Part model, mm, in its own coordinate system. Face numbers are marked on the shaded views. A direction names the side the tool comes from. Coordinates: 2 decimals unless noted, no trailing zeros. Order: outer loops, then holes, each group sorted by start corner. A loop starts at its lowest first (then second) coordinate and runs counter-clockwise, first axis right, second up. Notation, with made-up numbers: M -30,40 L -17,40 A31 ccw -17,79 Z; hole C 88,73.25 d11. An arc over 180 degrees is marked long. Write item = value, one per line. Start each with the question number.
from build123d import *

# Parameters (mm, degrees)
BASE_FLANGE1_DEPTH      = 44
CUT_EXTRUDE1_DEPTH      = 57
CUT_EXTRUDE1_DEPTH_BACK = 42
SKETCH7_R               = 4
CUT_EXTRUDE2_DEPTH      = 42
SKETCH8_R               = 7.25
CUT_EXTRUDE3_DEPTH      = 42
SKETCH9_W               = 2.5
SKETCH9_H               = 6
CUT_EXTRUDE4_DEPTH      = 13


# Sheet-metal steps are written as plain solids
with BuildPart() as part:
    # Sketch1 → Base-Flange1 (new body)
    with BuildSketch(Plane.XY):
        with BuildLine():
            Line((15, 0), (15, 73.75))
            ThreePointArc((15, 73.75), (14.121320344, 75.871320344), (12, 76.75))
            Line((12, 76.75), (-12, 76.75))
            ThreePointArc((-12, 76.75), (-14.121320344, 75.871320344), (-15, 73.75))
            Line((-15, 73.75), (-15, 0))
            Line((-15, 0), (-17.3, 0))
            Line((-17.3, 0), (-17.3, 73.75))
            ThreePointArc((-17.3, 73.75), (-15.74766594, 77.49766594), (-12, 79.05))
            Line((-12, 79.05), (12, 79.05))
            ThreePointArc((12, 79.05), (15.74766594, 77.49766594), (17.3, 73.75))
            Line((17.3, 73.75), (17.3, 0))
            Line((17.3, 0), (15, 0))
        make_face()
    extrude(amount=BASE_FLANGE1_DEPTH)

    # Sketch6 → Cut-Extrude1 (cut, two sides: drawn at the far end of the back side and taken through both)
    with BuildSketch(Plane(origin=(0, 0, 0), x_dir=(0, 0, -1), z_dir=(1, 0, 0)).offset(-CUT_EXTRUDE1_DEPTH_BACK)):
        with BuildLine():
            Line((0, 73.75), (-24.610061631, 6.560660321))
            ThreePointArc((-24.610061631, 6.560660321), (-35.746513142, 0.153696539), (-44, 10))
            Line((-44, 10), (-44, 36.875))
            Line((-44, 36.875), (-75.735832134, 36.875))
            Line((-75.735832134, 36.875), (-75.735832134, -15.470238138))
            Line((-75.735832134, -15.470238138), (20.414497878, -15.470238138))
            Line((20.414497878, -15.470238138), (20.414497878, 73.75))
            Line((20.414497878, 73.75), (0, 73.75))
        make_face()
    extrude(amount=CUT_EXTRUDE1_DEPTH + CUT_EXTRUDE1_DEPTH_BACK, mode=Mode.SUBTRACT)

    # Sketch7 → Cut-Extrude2 (cut)
    with BuildSketch(Plane(origin=(17.3, 0, 0), x_dir=(0, 0, -1), z_dir=(1, 0, 0))):
        with Locations(Location((-34, 10, 0), (0, 0, 90))):
            Circle(SKETCH7_R)
    extrude(amount=-CUT_EXTRUDE2_DEPTH, mode=Mode.SUBTRACT)

    # Sketch8 → Cut-Extrude3 (cut)
    with BuildSketch(Plane(origin=(0, 79.05, 0), x_dir=(1, 0, 0), z_dir=(0, 1, 0))):
        with Locations(Location((0, -22, 0), (0, 0, 270))):
            Circle(SKETCH8_R)
    extrude(amount=-CUT_EXTRUDE3_DEPTH, mode=Mode.SUBTRACT)

    # Sketch9 → Cut-Extrude4 (cut)
    with BuildSketch(Plane.ZY.offset(17.3)):
        with Locations((34, 13)):
            Rectangle(SKETCH9_W, SKETCH9_H)
    extrude(amount=-CUT_EXTRUDE4_DEPTH, mode=Mode.SUBTRACT)


solid = part.part
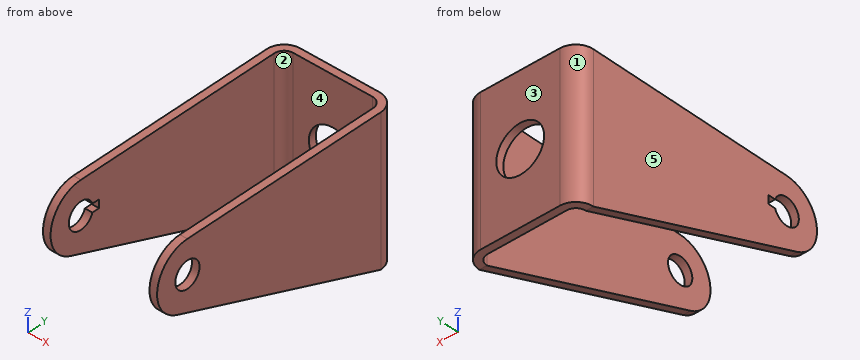
Item 1: 3-axis set-ups, long thin cutter, end or side, ignore diameter. For the marked faces 1 and 2: which of +Z, -Z, +X, -X, +Y, -Y reach the whole face in a straight line?
Item 2: Pull direction X, two halves, no side cores. Call the marked faces 3, 4 and 5: pulls with the +X half, pulls with the -X half, needs draft (parallel to the pull), parting line crosses it, or undercut.
Item 3: Wall check: line 1 along X through (y, z) = (37.5, 37.5); line 2 along Y through (x, z) = (8.5, 38.5); line 3 along Z through (x, y) = (-16.5, 10). Give the ranges that are in metal, low to high. Write a range as [from, to].
Item 4: Cut at D-D, the plane z = 22.5. Write the cut outline in (x, y).
Item 5: Cut at A-A, the plane x = 0. Write the cut outline in (y, z), and give its area (4 significant figures).
Item 6: Flat gauge pins, fed straight in: pin 1 (1.5 mm diameter, centred on x = 13, z = 6.5, fed in from -Y); pin 2 (0.7 mm diameter, centred on x = -16.5, y = 15, fed in from -Z); pin 3 (12 mm diameter, centred on x = -3.5, z = 20, fed in from -Y). Where does each tip first touch, or does it go through?
Item 7: Cut at B-B, the plane z = 34. Write the cut outline in (x, y), and give its area (3 significant figures).
Item 8: Cut at C-C, the plane y = 37. Write the cut outline in (x, z).
Filled sheet:
q1.face_1 = +Z, -Z, -X, +Y
q1.face_2 = +Z, -Z, -Y
q2.face_3 = needs draft
q2.face_4 = undercut
q2.face_5 = pulls with the -X half
q3.line_1 = [-17.3, -15], [15, 17.3]
q3.line_2 = [76.75, 79.05]
q3.line_3 = [23.35, 30], [38, 44]
q4.outline = M -17.3,12.32 L -15,12.32 L -15,73.75 A3 cw -12,76.75 L -7.23,76.75 L -7.23,79.05 L -12,79.05 A5.3 ccw -17.3,73.75 Z; M 7.23,76.75 L 12,76.75 A3 cw 15,73.75 L 15,12.32 L 17.3,12.32 L 17.3,73.75 A5.3 ccw 12,79.05 L 7.23,79.05 Z
q5.outline = M 76.75,0 L 79.05,0 L 79.05,14.75 L 76.75,14.75 Z; M 76.75,29.25 L 79.05,29.25 L 79.05,44 L 76.75,44 Z
q5.area = 67.85 mm2
q6.pin_1 = 76.19
q6.pin_2 = 21.39
q6.pin_3 = 76.75
q7.outline = M -17.3,0 L -15,0 L -15,6 L -17.3,6 Z; M -17.3,16 L -15,16 L -15,73.75 A3 cw -12,76.75 L 12,76.75 A3 cw 15,73.75 L 15,14 L 17.3,14 L 17.3,73.75 A5.3 ccw 12,79.05 L -12,79.05 A5.3 ccw -17.3,73.75 Z; M 15,0 L 17.3,0 L 17.3,6 L 15,6 Z
q7.area = 383 mm2
q8.outline = M -17.3,13.46 L -15,13.46 L -15,44 L -17.3,44 Z; M 15,13.46 L 17.3,13.46 L 17.3,44 L 15,44 Z
